Check sheet for the drawn part. Datum: minimum x, y, z corner. Units: mm. Round coordinates to 2 decimals unless told otherwise and drop trailing zeros. Write each loop counter-clockwise with the first axis right and the second up, starting at its lowest first coordinate (ties: lowest second). Pieces come first, ordered by that corner, then holes.
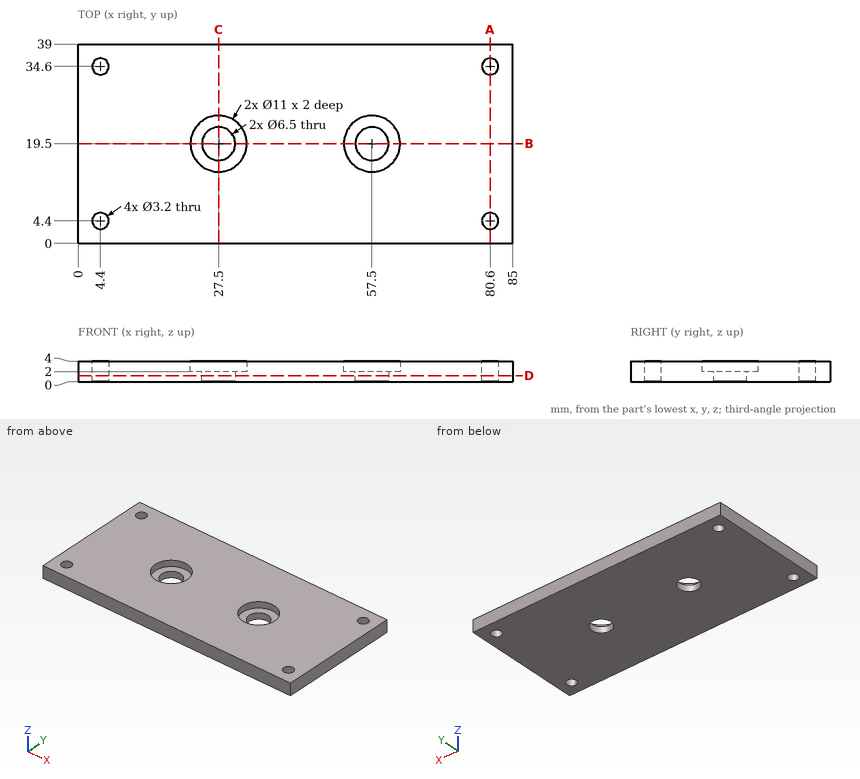
Q1. Sectioned sample at A-A (x = 80.6). Enter the section's corners in (y, z), plus the area to 3 significant figures.
Recorded:
outline: (0, 0) - (2.8, 0) - (2.8, 4) - (0, 4) - close; (6, 0) - (33, 0) - (33, 4) - (6, 4) - close; (36.2, 0) - (39, 0) - (39, 4) - (36.2, 4) - close
area: 130 mm2
Q2. Depth check by flat-ended pin: P1, Ø3.5, axis at x = 58, y = 20.5, coming from the +Z side; P2, Ø8.5, axis at x = 27.5, y = 19.5, coming from the +Z side. Enter the tip coordinate at first touch or a pass-through.
Recorded:
P1: passes through
P2: stops at z = 2
Q3. Sectioned sample at C-C (x = 27.5). Enter the section's corners in (y, z).
Recorded:
outline: (0, 0) - (16.25, 0) - (16.25, 2) - (14, 2) - (14, 4) - (0, 4) - close; (22.75, 0) - (39, 0) - (39, 4) - (25, 4) - (25, 2) - (22.75, 2) - close
Q4. Sectioned sample at D-D (z = 1.2). Enter the section's corners in (x, y).
Recorded:
outline: (0, 0) - (85, 0) - (85, 39) - (0, 39) - close; hole circle Ø3.2 at (4.4, 4.4); hole circle Ø3.2 at (4.4, 34.6); hole circle Ø6.5 at (27.5, 19.5); hole circle Ø6.5 at (57.5, 19.5); hole circle Ø3.2 at (80.6, 4.4); hole circle Ø3.2 at (80.6, 34.6)
Q5. Material ranges on line 1 along Y through (x, z) = (80.6, 1.6); line 2 along Y through (x, z) = (57.5, 0.4); line 3 along Y through (x, z) = (27.5, 3.05), recorded low to high.
Recorded:
line 1: y = 0 to 2.8, 6 to 33, 36.2 to 39
line 2: y = 0 to 16.25, 22.75 to 39
line 3: y = 0 to 14, 25 to 39
Q6. Sectioned sample at B-B (y = 19.5). Enter the section's corners in (x, z).
Recorded:
outline: (0, 0) - (24.25, 0) - (24.25, 2) - (22, 2) - (22, 4) - (0, 4) - close; (30.75, 0) - (54.25, 0) - (54.25, 2) - (52, 2) - (52, 4) - (33, 4) - (33, 2) - (30.75, 2) - close; (60.75, 0) - (85, 0) - (85, 4) - (63, 4) - (63, 2) - (60.75, 2) - close
